Job drawing, mm, ordinate dimensions from the low corner. One solid piece. Coordinates: 2 decimals unless noted, no trailing zeros.
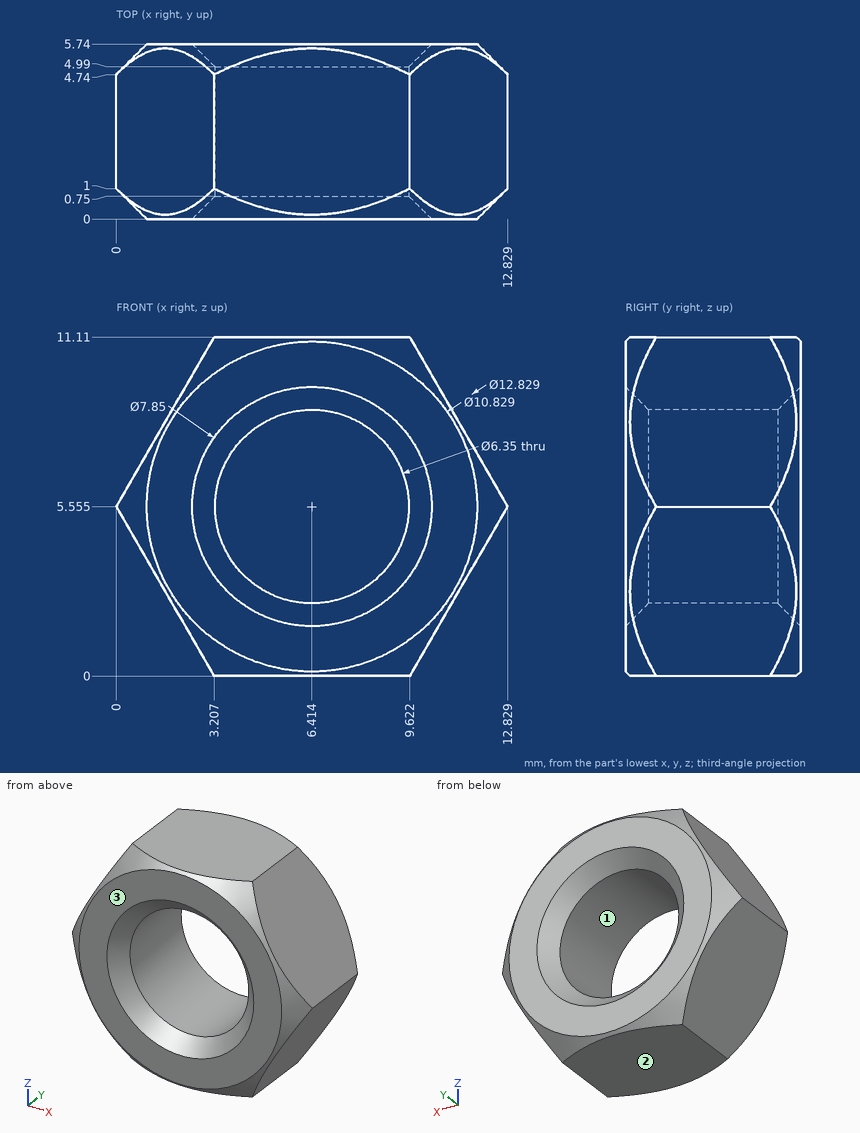
1. Flat gauge pin, fed straight in: pin 1 (1 mm diameter, centred on y = 4.5, z = 4, fed in from -X). Where does the tip first touch, or does it go through?
Computed values:
pin 1: stops at x = 0.61
2. Probe line 1 along X through (y, z) = (3.7, 1.25) (1 decimal); line 2 along Z through (x, y) = (6.25, 4.6) (1 decimal); line 3 along X through (y, z) = (3.15, 4.5). List the from-to ranges inside material, lowest first.
Computed values:
line 1: x = 2.5 to 10.3
line 2: z = 0 to 2.4, 8.7 to 11.1
line 3: x = 0.61 to 3.42, 9.41 to 12.22
3. Mould opens along Z. For the marked faces 1, 2 and 3 say: +Z half, -Z half, draft (parallel to the pull), parting line (faces both ways), or undercut.
Computed values:
face 1: undercut
face 2: -Z half
face 3: draft
